The model under review builds one solid part; all positions refer to its coordinate system, in mm. Face numbers are marked on the shaded views. A direction names the side the tool comes from. Give positions to 0.01 mm unless a question says otherwise; leave off trailing zeros. Loops run counter-clockwise (first coordinate to the right, second up) from the corner with the lowest first, then second, coordinate; pieces in that order, holes last. Notation, with made-up numbers: (-1.5, -29.5) - (4.5, -29.5) arc R10 ccw to (4.5, -17.5) - close; hole circle Ø5 at (-25.75, 61). An arc over 180 degrees is marked (long way). Return JSON: item names as keys, results as strings. Group by question number.
from build123d import *

# Parameters (mm, degrees)
F1_DEPTH       = 76.2
F3_DEPTH       = 35.561
F7_D           = 7.62
F7_DEPTH       = 27.94
F7_TIP         = 2.2892789585
F8_DEPTH       = 27.94
F9_D           = 15.24
F9_CBORE_D     = 40.64
F9_CBORE_DEPTH = 10.16
F10_DEPTH      = 10.16
F4_R           = 10.16
F11_DEPTH      = 76.201


with BuildPart() as f1:
    # F0 (on Right) → F1 (new body)
    with BuildSketch(Plane.YZ):
        Polygon((0, 35.56), (0, 0), (111.76, 0), (147.32, 35.56), (147.32, 71.12), (111.76, 71.12), (76.2, 35.56), align=None)
    extrude(amount=F1_DEPTH)

    # F2 (on face) → F3 (cut, through all)
    with BuildSketch(Plane.XY.offset(35.56)):
        with BuildLine():
            Line((0, 0), (10.16, 0))
            ThreePointArc((10.16, 0), (2.9757951031, 2.9757951031), (0, 10.16))
            Line((0, 10.16), (0, 0))
        make_face()
        with BuildLine():
            ThreePointArc((76.2, 10.16), (73.2242048969, 2.9757951031), (66.04, 0))
            Line((66.04, 0), (76.2, 0))
            Line((76.2, 0), (76.2, 10.16))
        make_face()
    extrude(amount=-F3_DEPTH, mode=Mode.SUBTRACT)

    # F7
    with Locations(Plane.XY.offset(71.12)):
        with Locations((15.24, 129.54), (60.96, 129.54)):
            Hole(F7_D / 2, depth=F7_DEPTH)
            with Locations((0, 0, -(F7_DEPTH + F7_TIP / 2))):  # 118° drill point
                Cone(0, F7_D / 2, F7_TIP, mode=Mode.SUBTRACT)

    # F5 (on face) → F8 (cut)
    with BuildSketch(Plane.XY.offset(71.12)):
        with BuildLine():
            ThreePointArc((15.24, 133.35), (11.43, 129.54), (15.24, 125.73))
            Line((15.24, 125.73), (60.96, 125.73))
            ThreePointArc((60.96, 125.73), (64.77, 129.54), (60.96, 133.35))
            Line((60.96, 133.35), (15.24, 133.35))
        make_face()
    extrude(amount=-F8_DEPTH, mode=Mode.SUBTRACT)

    # F9 (through all)
    with Locations(Plane.XY.offset(35.56)):
        with Locations((38.1, 38.1)):
            CounterBoreHole(F9_D / 2, F9_CBORE_D / 2, F9_CBORE_DEPTH)

    # F6 (on face) → F10 (cut)
    with BuildSketch(Plane.XY.offset(35.56)):
        with BuildLine():
            Line((43.18, 0), (43.18, 32.4203873372))
            ThreePointArc((43.18, 32.4203873372), (38.1, 30.48), (33.02, 32.4203873372))
            Line((33.02, 32.4203873372), (33.02, 0))
            Line((33.02, 0), (43.18, 0))
        make_face()
        with BuildLine():
            ThreePointArc((33.02, 43.7796126628), (38.1, 45.72), (43.18, 43.7796126628))
            Line((43.18, 43.7796126628), (43.18, 76.2))
            Line((43.18, 76.2), (33.02, 76.2))
            Line((33.02, 76.2), (33.02, 43.7796126628))
        make_face()
    extrude(amount=-F10_DEPTH, mode=Mode.SUBTRACT)

    # F4 (on face) → F11 (cut, through all)
    with BuildSketch(Plane.YZ.offset(76.2)):
        with Locations((93.98, 20.32)):
            Circle(F4_R)
    extrude(amount=-F11_DEPTH, mode=Mode.SUBTRACT)


solid = f1.part
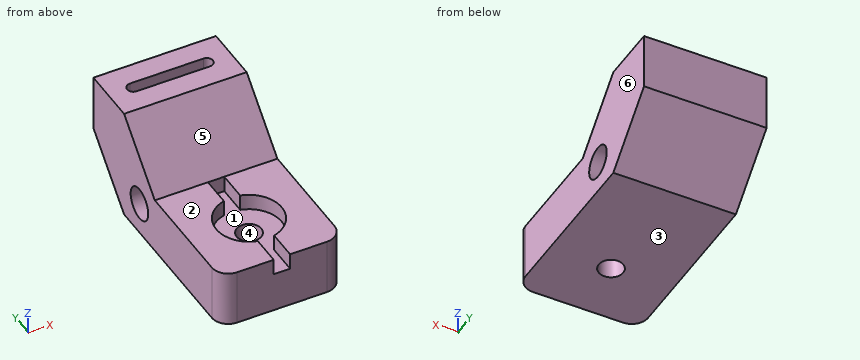
Item 1: For P1, Ø3, axis at x = 36, z = 28, coming from the -Y side; P2, Ø1, axis at x = 21.5, y = 32.5, coming from the -Z side; P3, Ø8.5, axis at x = 41.5, z = 53.5, coming from the -Y side; P4, Ø1.5, axis at x = 8.5, z = 45, coming from the -Y side, all flat-tipped, find the tip position at first contact; note any pin that passes through.
Item 2: Take a section at B-B (y = 93.98). State the section outline as (x, z) points.
Item 3: Tool access review of the marked faces 1, 2 and 3: name each direction out of +Z, -Z, +X, -X, +Y, -Y from which nothing blocks a thin tool from reaching the whole face with its end or side.
Item 4: Take a section at D-D (z = 28.5). State the section outline as (x, y) points.
Item 5: Mouldability with a two-part tool opening along Y and no side actions: class the marked faces 4, 5 and 6 as +Y half, -Y half, draft (parallel to the pull), parting line (faces both ways), or undercut.
Item 6: Take a section at C-C (z = 12). State the section outline as (x, y) points, then the cut area to 3 significant figures.
Item 7: Take a section at A-A (x = 38.1). State the section outline as (y, z) points.
Item 8: For L1, parallel to X at y = 38.1, z = 16.5; L2, parallel to Z at x = 14.5, y = 38; L3, parallel to Z at x = 34.5, y = 93.98, list the stretches that pass through material, from the lowest coordinate up. Write a range as from..to.
Check sheet entries:
{
 "1": {"P1": "stops at y = 76.2", "P2": "stops at z = 0", "P3": "stops at y = 89.89", "P4": "stops at y = 84.89"},
 "2": {"outline": "(0, 0) - (76.2, 0) - (76.2, 10.16) - (0, 10.16) - close; (0, 30.48) - (76.2, 30.48) - (76.2, 53.34) - (0, 53.34) - close"},
 "3": {"face 1": "+Z", "face 2": "+Z, +X, -X, -Y", "face 3": "-Z, +X, -X, +Y, -Y"},
 "4": {"outline": "(0, 10.16) arc R10.16 ccw to (10.16, 0) - (33.02, 0) - (33.02, 18.43) arc R20.32 cw to (33.02, 57.77) - (33.02, 76.2) - (43.18, 76.2) - (43.18, 57.77) arc R20.32 cw to (43.18, 18.43) - (43.18, 0) - (66.04, 0) arc R10.16 ccw to (76.2, 10.16) - (76.2, 87.95) - (0, 87.95) - close; (0, 100.01) - (76.2, 100.01) - (76.2, 140.26) - (0, 140.26) - close"},
 "5": {"face 4": "undercut", "face 5": "-Y half", "face 6": "draft"},
 "6": {"outline": "(0, 10.16) arc R10.16 ccw to (10.16, 0) - (66.04, 0) arc R10.16 ccw to (76.2, 10.16) - (76.2, 88.15) - (0, 88.15) - close; (0, 99.81) - (76.2, 99.81) - (76.2, 123.76) - (0, 123.76) - close; hole circle Ø15.24 at (38.1, 38.1)", "area": "8,320 mm^2"},
 "7": {"outline": "(0, 0) - (30.48, 0) - (30.48, 25.4) - (0, 25.4) - close; (45.72, 0) - (111.76, 0) - (147.32, 35.56) - (147.32, 71.12) - (133.35, 71.12) - (133.35, 43.18) - (125.73, 43.18) - (125.73, 71.12) - (111.76, 71.12) - (76.2, 35.56) - (76.2, 25.4) - (45.72, 25.4) - close; hole circle Ø20.32 at (93.98, 20.32)"},
 "8": {"L1": "x = 0..30.48, 45.72..76.2", "L2": "z = 0..35.56", "L3": "z = 0..10.16, 30.48..53.34"}
}
